Can you work these out from the model? Positions are in its coordinate system, mm. A direction names the side the tool comes from. Give positions to 0.01 mm unless a question says otherwise; leave off trailing zeros. Loops run counter-clockwise (first coordinate to the right, second up) from the corner with the lowest first, then second, coordinate; pieces in that order, holes last. Notation, with made-up numbers: (32.25, 28.5) - (52.25, 28.5) arc R26 ccw to (52.25, 54.5) - close; hole circle Ø6 at (-5, -4). An arc over 180 degrees is marked (long way). Answer as a JSON object with one key per item and string values. Group by question number.
Item 1: Which directions (+Z, -Z, +X, -X, +Y, -Y) give clear straight access to the entire face, cutting with the end or side of a thin tool? Please do faces 1 (the flat face through (24, 2, 4.55)), 2 (the conical face through (1.115, 14.533, 2.242)).
Item 2: Suppose I cut it at A-A on y = 16.5. Write out the boundary of the cut face in (x, z).
Item 3: Will these pins go through, and if not, where does the flat tip stop? pin 1 (1.8 mm diameter, centred on x = 48.01, y = 31.2, fed in from +Z); pin 2 (4 mm diameter, centred on x = 2.5, y = 17.5, fed in from +Z); pin 3 (1.5 mm diameter, centred on y = 21, z = 3, fed in from -X); pin 4 (2 mm diameter, centred on x = 16.5, y = 1.5, fed in from +Z).
Item 4: Thinking about a two-plate mould opening in Y: for faces 3 (the flat face through (24, 0, 2)), 4 (the conical face through (1.09, 18.09, 2.24)), 5 (the flat face through (24, 16, 0)), 6 (the flat face through (24, 32.4, 2)), which applies, pulls with the +Y half, pulls with the -Y half, needs draft (parallel to the pull), parting line crosses it, or undercut?
Item 5: Suppose I cut it at B-B on z = 3.7. Write out the boundary of the cut face in (x, y), and give its area (3 significant figures).
Item 6: Please list where these lines run through material, in increasing order: L1, parallel to X at y = 30.5, z = 4.2; L2, parallel to Z at x = 3.5, y = 18; L3, parallel to Z at x = 29, y = 2.5.
from build123d import *

# Parameters (mm, degrees)
ESQUISSE1_W             = 49.4
ESQUISSE1_H             = 32.4
BOSS_EXTRU_1_DEPTH      = 1.6
ESQUISSE5_W             = 42.06
ESQUISSE5_H             = 32.4
BOSS_EXTRU_2_DEPTH      = 3
ESQUISSE6_R             = 0.8
ENL_V_MAT_EXTRU_1_DEPTH = 3
ESQUISSE7_W             = 42.06
ESQUISSE7_H             = 4.035624865
ENL_V_MAT_EXTRU_2_DEPTH = 0.05
ESQUISSE8_R             = 0.6
BOSS_EXTRU_3_DEPTH      = 1.2
BOSS_EXTRU_3_TAPER      = 30


with BuildPart() as part:
    # Esquisse1 → Boss.-Extru.1 (new body)
    with BuildSketch(Plane.XY):
        with Locations((24.7, 16.2)):
            Rectangle(ESQUISSE1_W, ESQUISSE1_H)
    extrude(amount=BOSS_EXTRU_1_DEPTH)

    # Esquisse5 → Boss.-Extru.2 (add)
    with BuildSketch(Plane.XY.offset(1.6)):
        with Locations((24.7, 16.2)):
            Rectangle(ESQUISSE5_W, ESQUISSE5_H)
    extrude(amount=BOSS_EXTRU_2_DEPTH)

    # Esquisse6 → Enlèv. mat.-Extru.1 (cut)
    with BuildSketch(Plane.XY.offset(1.6)):
        with Locations((1.144377661, 31.203769118)):
            Circle(ESQUISSE6_R)
        with Locations((1.144377661, 1.31386178)):
            Circle(ESQUISSE6_R)
        with Locations((48.008189331, 1.31386178)):
            Circle(ESQUISSE6_R)
        with Locations((48.008189331, 31.203769118)):
            Circle(ESQUISSE6_R)
    extrude(amount=-ENL_V_MAT_EXTRU_1_DEPTH, mode=Mode.SUBTRACT)

    # Esquisse7 → Enlèv. mat.-Extru.2 (cut)
    with BuildSketch(Plane.XY.offset(4.6)):
        with Locations((24.7, 2.017812432)):
            Rectangle(ESQUISSE7_W, ESQUISSE7_H)
    extrude(amount=-ENL_V_MAT_EXTRU_2_DEPTH, mode=Mode.SUBTRACT)

    # Esquisse8 → Boss.-Extru.3 (add)
    with BuildSketch(Plane.XY.offset(1.6)):
        with Locations((1.144377661, 21.803769118)):
            Circle(ESQUISSE8_R)
        with Locations((1.144377661, 10.71386178)):
            Circle(ESQUISSE8_R)
        with Locations((48.008189331, 21.803769118)):
            Circle(ESQUISSE8_R)
        with Locations((48.008189331, 10.71386178)):
            Circle(ESQUISSE8_R)
        with Locations((1.144377661, 18.315710158)):
            Circle(ESQUISSE8_R)
        with Locations((1.144377661, 14.305919008)):
            Circle(ESQUISSE8_R)
        with Locations((48.008189331, 18.315710158)):
            Circle(ESQUISSE8_R)
        with Locations((48.008189331, 14.305919008)):
            Circle(ESQUISSE8_R)
    extrude(amount=BOSS_EXTRU_3_DEPTH, taper=BOSS_EXTRU_3_TAPER)


solid = part.part
Worked out:
{
 "1": {"face 1": "+Z, +X, -X, -Y", "face 2": "+Z"},
 "2": {"outline": "(0, 0) - (49.4, 0) - (49.4, 1.6) - (45.73, 1.6) - (45.73, 4.6) - (3.67, 4.6) - (3.67, 1.6) - (0, 1.6) - close"},
 "3": {"pin 1": "stops at z = 1.6", "pin 2": "stops at z = 4.6", "pin 3": "stops at x = 3.67", "pin 4": "stops at z = 4.55"},
 "4": {"face 3": "pulls with the -Y half", "face 4": "undercut", "face 5": "needs draft", "face 6": "pulls with the +Y half"},
 "5": {"outline": "(3.67, 0) - (45.73, 0) - (45.73, 32.4) - (3.67, 32.4) - close", "area": "1,360 mm2"},
 "6": {"L1": "x = 3.67 to 45.73", "L2": "z = 0 to 1.6", "L3": "z = 0 to 4.55"}
}
